Could you check a few things on this model? Use its own coordinates, in mm. Face numbers are marked on the shaded views. A direction names the side the tool comes from. Give positions to 0.01 mm unless a question says otherwise; leave off trailing zeros. Loops run counter-clockwise (first coordinate to the right, second up) from the corner with the lowest first, then second, coordinate; pieces in that order, holes last. Notation, with made-up numbers: M 55.25,-23 L 73.25,-23 A25 cw 73.25,9 Z; hole C -26,57.5 d11. An arc over 180 degrees is marked long. Use CSV: the item, a comma, the result in double quotes.
```python
from build123d import *

# Parameters (mm, degrees)
SKETCH3_W           = 86
SKETCH3_H           = 86
BOSS_EXTRUDE1_DEPTH = 6
FILLET2_R           = 2
BOSS_EXTRUDE2_START = 43
SKETCH4_R           = 11
BOSS_EXTRUDE2_DEPTH = 86
SKETCH4_2_R         = 11
CUT_EXTRUDE1_DEPTH  = 36
CHAMFER2_SIZE       = 2


with BuildPart() as part:
    # Sketch2 → Revolve1 (revolve)
    with BuildSketch(Plane.XY, mode=Mode.PRIVATE) as revolve1_sk:
        Polygon((0, 0), (15.5, 0), (14.10316922, -40), (0, -40), align=None)
    revolve(revolve1_sk.sketch.rotate(Axis((0, -16.883928571, 0), (0, 1, 0)), 90), axis=Axis((0, -16.883928571, 0), (0, 1, 0)))

    # Sketch3 → Boss-Extrude1 (add)
    with BuildSketch(Plane(origin=(0, 0, 0), x_dir=(1, 0, 0), z_dir=(0, 1, 0))):
        Rectangle(SKETCH3_W, SKETCH3_H)
    extrude(amount=BOSS_EXTRUDE1_DEPTH)

    # Fillet2
    fillet2_edges = [part.edges().sort_by_distance(p)[0] for p in [
        (0, 0, 15.5),
    ]]
    fillet(fillet2_edges, radius=FILLET2_R)

    # Sketch4 → Boss-Extrude2 (add)
    with BuildSketch(Plane(origin=(0, 0, 0), x_dir=(0, 0, -1), z_dir=(1, 0, 0)).offset(BOSS_EXTRUDE2_START)):
        with BuildLine():
            Line((-43, 6), (43, 6))
            Line((43, 6), (43, 32))
            ThreePointArc((43, 32), (0, 75), (-43, 32))
            Line((-43, 32), (-43, 6))
        make_face()
        with Locations((0, 32)):
            Circle(SKETCH4_R, mode=Mode.SUBTRACT)
    extrude(amount=-BOSS_EXTRUDE2_DEPTH)

    # Sketch4<2> → Cut-Extrude1 (cut, symmetric)
    with BuildSketch(Plane(origin=(0, 0, 0), x_dir=(0, 0, -1), z_dir=(1, 0, 0))):
        with BuildLine():
            Line((-43, 6), (43, 6))
            Line((43, 6), (43, 32))
            ThreePointArc((43, 32), (0, 75), (-43, 32))
            Line((-43, 32), (-43, 6))
        make_face()
        with Locations((0, 32)):
            Circle(SKETCH4_2_R, mode=Mode.SUBTRACT)
    extrude(amount=CUT_EXTRUDE1_DEPTH, both=True, mode=Mode.SUBTRACT)

    # Chamfer2
    chamfer2_edges = [part.edges().sort_by_distance(p)[0] for p in [
        (0, 6, 43),
    ]]
    chamfer(chamfer2_edges, length=CHAMFER2_SIZE)


solid = part.part
```
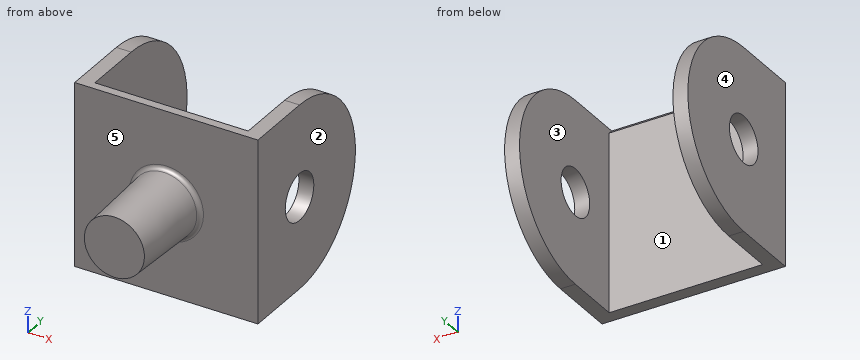
1. I want a section at D-D, the plane x = -28.5. List the corners of the cut face in (y, z) for me, then the cut area to 3 significant figures.
Outcome:
outline,"M 0,-43 L 6,-43 L 6,41 L 4,43 L 0,43 Z"
area,"514 mm2"
2. I want a section at C-C, the plane z = 34.5. List the corners of the cut face in (x, y) for me.
Outcome:
outline,"M -43,0 L 43,0 L 43,57.67 L 36,57.67 L 36,6 L -36,6 L -36,57.67 L -43,57.67 Z"
3. I want a section at A-A, the plane z = 0. List the corners of the cut face in (x, y) for me, then the cut area to 3 significant figures.
Outcome:
outline,"M -43,0 L -17.43,0 A2 cw -15.43,-1.93 L -14.1,-40 L 14.1,-40 L 15.43,-1.93 A2 cw 17.43,0 L 43,0 L 43,21 L 36,21 L 36,6 L -36,6 L -36,21 L -43,21 Z; M -43,43 L -36,43 L -36,75 L -43,75 Z; M 36,43 L 43,43 L 43,75 L 36,75 Z"
area,"2,360 mm2"
4. I want a section at B-B, the plane y = 37.5. List the corners of the cut face in (x, z) for me, then the cut area to 3 significant figures.
Outcome:
outline,"M -43,-42.65 L -36,-42.65 L -36,-9.53 L -43,-9.53 Z; M -43,9.53 L -36,9.53 L -36,42.65 L -43,42.65 Z; M 36,-42.65 L 43,-42.65 L 43,-9.53 L 36,-9.53 Z; M 36,9.53 L 43,9.53 L 43,42.65 L 36,42.65 Z"
area,"927 mm2"
5. I'm going to push flat-ended pins straight in: pin 1 Ø3 at (x, z) = (-25.5, 25.5) entering from -Y; pin 2 Ø10 at (x, y) = (2, -9.5) entering from +Z; pin 3 Ø5 at (x, z) = (11, 14.5) entering from -Y. Where does each tip first touch, or does it pass through?
Outcome:
pin 1,"y = 0"
pin 2,"z = 15.33"
pin 3,"y = -1"
6. If we mould it in two halves opening along X, with no side actions, what happens to the marked faces 3, 4 and 5? For each: +X half, -X half, draft (parallel to the pull), parting line (faces both ways), or undercut.
Outcome:
face 3,"undercut"
face 4,"-X half"
face 5,"draft"
7. Which directions (+Z, -Z, +X, -X, +Y, -Y) give clear straight access to the entire face, cutting with the end or side of a thin tool? Please do the marked faces 1 and 2.
Outcome:
face 1,"+Z, -Z, +Y"
face 2,"+Z, -Z, +X, +Y, -Y"
8. Please list where these lines run through material, in increasing order: line 1 (X direction, y = 15.5, z = 1.5); line 2 (Y direction, x = -38.5, z = 0); line 3 (Y direction, x = -25, z = -18).
Outcome:
line 1,"-43 to -36, 36 to 43"
line 2,"0 to 21, 43 to 75"
line 3,"0 to 6"
